Geometry check sheet. Reference: the model listing, model coordinates, mm. A direction names the side the tool comes from. Coordinates: 2 decimals unless noted, no trailing zeros. Loops run counter-clockwise (first coordinate to the right, second up) from the corner with the lowest first, then second, coordinate; pieces in that order, holes last. Notation, with made-up numbers: (75, 69) - (116, 69) arc R31 cw to (116, 103) - close; hole circle Ø9 at (-35.5, -6). An arc over 180 degrees is marked (long way). Write each question's results on one line, items separated by ' | '. Start each with the question number.
(1) Material ranges on probe 1 along X at (y, z) = (1.1, 13); probe 2 along Z at (x, y) = (25, 1.4); probe 3 along Z at (x, y) = (75, 1.7), recorded low to high.
(2) Access from +Z, -Z, +X, -X, +Y, -Y to the whole of each face (thin tool, end or side, straight path). Record for faces 1 (the face through (112, 0, 21)), 2 (the face through (68.775, 1.479, 42.262)).
(3) Mould release check, pull along X, two halves, no side actions. Record for faces 3 (the face through (112, 3, 21)), 4 (the face through (69.641, 1.479, 2.616)): pulls with the +X half, pulls with the -X half, needs draft (parallel to the pull), parting line crosses it, or undercut.
(4) Sectioned sample at A-A (z = 7). Enter the section's corners in (x, y), plus the area to 3 significant figures.
(5) Sectioned sample at D-D (x = 160.5). Enter the section's corners in (y, z), plus the area to 3 significant figures.
(6) Sectioned sample at C-C (x = 108.5). Enter the section's corners in (y, z), plus the area to 3 significant figures.
(7) Sectioned sample at B-B (y = 2.25). State how many separate pieces and enclosed holes the cut face has, plus the area to 3 significant figures.
(8) Go/stop test with a flat-tipped pin: pin 1 Ø2.5 at (x, z) = (221.79, 67.7) entering from -Y. Record where the tip stops, or that it passes through.
from build123d import *

# Parameters (mm, degrees)
SKETCH_1_W      = 229
SKETCH_1_H      = 115
SKETCH_1_R      = 1.5
EXTRUDE_6_DEPTH = 3


with BuildPart() as part:
    # 草图1 → 凸台-拉伸6 (new body)
    with BuildSketch(Plane(origin=(0, 0, 0), x_dir=(1, 0, 0), z_dir=(0, 1, 0))):
        with Locations((113.28975623, -22.19835875)):
            Rectangle(SKETCH_1_W, SKETCH_1_H)
        with Locations(Location((25.78975623, 23.30164125, 0), (0, 0, 270))):
            Circle(SKETCH_1_R, mode=Mode.SUBTRACT)
        with Locations(Location((25.78975623, -67.69835875, 0), (0, 0, 270))):
            Circle(SKETCH_1_R, mode=Mode.SUBTRACT)
        with Locations(Location((221.78975623, 23.30164125, 0), (0, 0, 270))):
            Circle(SKETCH_1_R, mode=Mode.SUBTRACT)
        with Locations(Location((221.78975623, -67.69835875, 0), (0, 0, 270))):
            Circle(SKETCH_1_R, mode=Mode.SUBTRACT)
        with BuildLine():
            Line((49.910205521, 17.679169422), (111.832827436, -16.722287198))
            ThreePointArc((111.832827436, -16.722287198), (113.28975623, -17.099815369), (114.746685023, -16.722287198))
            Line((114.746685023, -16.722287198), (176.669306939, 17.679169422))
            ThreePointArc((176.669306939, 17.679169422), (178.11646281, 21.054165175), (175.212378145, 23.30164125))
            Line((175.212378145, 23.30164125), (51.367134314, 23.30164125))
            ThreePointArc((51.367134314, 23.30164125), (48.463049649, 21.054165175), (49.910205521, 17.679169422))
        make_face(mode=Mode.SUBTRACT)
        with BuildLine():
            Line((192.78975623, 12.20309787), (192.78975623, -56.599815369))
            ThreePointArc((192.78975623, -56.599815369), (191.311139419, -59.185428099), (188.332827436, -59.222287198))
            Line((188.332827436, -59.222287198), (126.410205521, -24.820830578))
            ThreePointArc((126.410205521, -24.820830578), (124.867134314, -22.19835875), (126.410205521, -19.575886921))
            Line((126.410205521, -19.575886921), (188.332827436, 14.825569699))
            ThreePointArc((188.332827436, 14.825569699), (191.311139419, 14.7887106), (192.78975623, 12.20309787))
        make_face(mode=Mode.SUBTRACT)
        with BuildLine():
            Line((114.746685023, -27.674430301), (176.669306939, -62.075886921))
            ThreePointArc((176.669306939, -62.075886921), (178.11646281, -65.450882674), (175.212378145, -67.69835875))
            Line((175.212378145, -67.69835875), (51.367134314, -67.69835875))
            ThreePointArc((51.367134314, -67.69835875), (48.463049649, -65.450882674), (49.910205521, -62.075886921))
            Line((49.910205521, -62.075886921), (111.832827436, -27.674430301))
            ThreePointArc((111.832827436, -27.674430301), (113.28975623, -27.29690213), (114.746685023, -27.674430301))
        make_face(mode=Mode.SUBTRACT)
        with BuildLine():
            Line((100.169306939, -19.575886921), (38.246685023, 14.825569699))
            ThreePointArc((38.246685023, 14.825569699), (35.26837304, 14.7887106), (33.78975623, 12.20309787))
            Line((33.78975623, 12.20309787), (33.78975623, -56.599815369))
            ThreePointArc((33.78975623, -56.599815369), (35.26837304, -59.185428099), (38.246685023, -59.222287198))
            Line((38.246685023, -59.222287198), (100.169306939, -24.820830578))
            ThreePointArc((100.169306939, -24.820830578), (101.712378145, -22.19835875), (100.169306939, -19.575886921))
        make_face(mode=Mode.SUBTRACT)
    extrude(amount=EXTRUDE_6_DEPTH)


solid = part.part
Outcome:
1) probe 1: x = -1.21 to 33.79, 88.33 to 105.13, 121.45 to 138.25, 192.79 to 227.79 | probe 2: z = -35.3 to -24.58, -22.03 to 66.42, 68.97 to 79.7 | probe 3: z = -35.3 to -23.3, -3.74 to 5.59, 38.8 to 48.14, 67.7 to 79.7
2) face 1: +Z, -Z, +X, -X, -Y | face 2: +Y, -Y
3) face 3: needs draft | face 4: undercut
4) outline: (-1.21, 0) - (33.79, 0) - (33.79, 3) - (-1.21, 3) - close; (77.53, 0) - (94.33, 0) - (94.33, 3) - (77.53, 3) - close; (132.25, 0) - (149.05, 0) - (149.05, 3) - (132.25, 3) - close; (192.79, 0) - (227.79, 0) - (227.79, 3) - (192.79, 3) - close | area: 311 mm2
5) outline: (0, -35.3) - (3, -35.3) - (3, -23.3) - (0, -23.3) - close; (0, -8.7) - (3, -8.7) - (3, 0.64) - (0, 0.64) - close; (0, 43.76) - (3, 43.76) - (3, 53.09) - (0, 53.09) - close; (0, 67.7) - (3, 67.7) - (3, 79.7) - (0, 79.7) - close | area: 128 mm2
6) outline: (0, -35.3) - (3, -35.3) - (3, -23.3) - (0, -23.3) - close; (0, 14.87) - (3, 14.87) - (3, 29.53) - (0, 29.53) - close; (0, 67.7) - (3, 67.7) - (3, 79.7) - (0, 79.7) - close | area: 116 mm2
7) separate pieces: 1 | enclosed holes: 8 | area: 14,800 mm2
8) pin 1: passes through
